Verification items for this drawing (mm, ordinates from the low corner). A direction names the side the tool comes from. Give positions to 0.01 mm unless a question says otherwise; leave off trailing zeros. Loops run counter-clockwise (first coordinate to the right, second up) from the corner with the lowest first, then second, coordinate; pieces in that order, holes last. Notation, with made-up numbers: (77, 55.5) -> (88, 55.5) arc R19 cw to (88, 76.5) -> close; hole circle Ø8 at (-6.5, 75.5). An arc over 180 degrees is marked (long way). Write each question's results on one line, items separated by ' | '. Start each with the question number.
1) Scan lines: line 1 (X direction, y = 4.85, z = 46); line 2 (Z direction, x = 83, y = 4.4); line 3 (X direction, y = 20, z = 12). Record each from-to range of solid material in increasing order. Write a range as from..to.
2) Sectioned sample at A-A on z = 4. Record the cut outline in (x, y), then the cut area to 3 significant figures.
3) Set-up check for the marked faces 1, 2, 3 and 4: record each of +Z, -Z, +X, -X, +Y, -Y from which the full face is reachable in a straight line by a thin tool's end or side.
4) Sectioned sample at B-B on x = 4. Record the cut outline in (y, z), then the cut area to 3 significant figures.
5) Sectioned sample at D-D on x = 55.5. Record the cut outline in (y, z), then the cut area to 3 significant figures.
6) Depth check by flat-ended pin: pin 1 (1 mm diameter, centred on x = 69.5, y = 4.5, fed in from -Z); pin 2 (3 mm diameter, centred on x = 85, z = 27, fed in from +Y); pin 3 (11 mm diameter, centred on x = 31.5, y = 30, fed in from -Z); pin 4 (3 mm diameter, centred on y = 8.5, z = 20.5, fed in from +X). Enter the tip coordinate at first touch or a pass-through.
7) Sectioned sample at C-C on z = 34. Record the cut outline in (x, y), then the cut area to 3 significant figures.
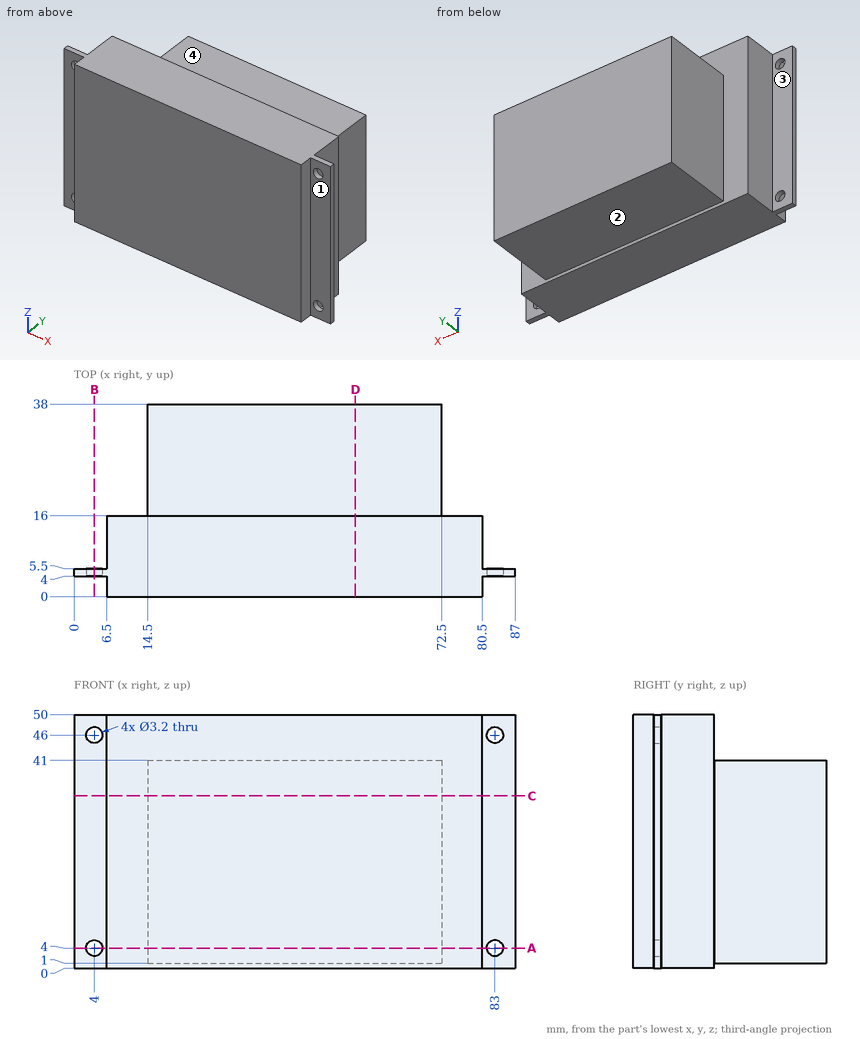
Result:
1) line 1: 0..2.4, 5.6..81.4, 84.6..87 | line 2: 0..2.4, 5.6..44.4, 47.6..50 | line 3: 14.5..72.5
2) outline: (0, 4) -> (2.4, 4) -> (2.4, 5.5) -> (0, 5.5) -> close; (5.6, 4) -> (6.5, 4) -> (6.5, 0) -> (80.5, 0) -> (80.5, 4) -> (81.4, 4) -> (81.4, 5.5) -> (80.5, 5.5) -> (80.5, 16) -> (72.5, 16) -> (72.5, 38) -> (14.5, 38) -> (14.5, 16) -> (6.5, 16) -> (6.5, 5.5) -> (5.6, 5.5) -> close; (84.6, 4) -> (87, 4) -> (87, 5.5) -> (84.6, 5.5) -> close | area: 2,470 mm^2
3) face 1: +Z, -Z, +X, -Y | face 2: -Z, +X, -X, +Y | face 3: +Z, -Z, -X, +Y | face 4: +Z, +X, -X, +Y
4) outline: (4, 0) -> (5.5, 0) -> (5.5, 2.4) -> (4, 2.4) -> close; (4, 5.6) -> (5.5, 5.6) -> (5.5, 44.4) -> (4, 44.4) -> close; (4, 47.6) -> (5.5, 47.6) -> (5.5, 50) -> (4, 50) -> close | area: 65.4 mm^2
5) outline: (0, 0) -> (16, 0) -> (16, 1) -> (38, 1) -> (38, 41) -> (16, 41) -> (16, 50) -> (0, 50) -> close | area: 1,680 mm^2
6) pin 1: z = 0 | pin 2: y = 5.5 | pin 3: z = 1 | pin 4: x = 80.5
7) outline: (0, 4) -> (6.5, 4) -> (6.5, 0) -> (80.5, 0) -> (80.5, 4) -> (87, 4) -> (87, 5.5) -> (80.5, 5.5) -> (80.5, 16) -> (72.5, 16) -> (72.5, 38) -> (14.5, 38) -> (14.5, 16) -> (6.5, 16) -> (6.5, 5.5) -> (0, 5.5) -> close | area: 2,480 mm^2
